from build123d import *

# Parameters (mm, degrees)
CHAMFER1_SIZE = 0.2


with BuildPart() as part:
    # Sketch1 → Revolve1 (revolve)
    with BuildSketch(Plane.XY, mode=Mode.PRIVATE) as revolve1_sk:
        Polygon((2.52, 0), (2.52, 4), (3.05, 4), (3.05, 6.4), (4.05, 6.4), (4.05, 4), (3.05, 0), align=None)
    revolve(revolve1_sk.sketch.rotate(Axis((0, 0, 0), (0, 1, 0)), 90), axis=Axis((0, 0, 0), (0, 1, 0)))

    # Chamfer1
    chamfer1_edges = [part.edges().sort_by_distance(p)[0] for p in [
        (0, 6.4, 3.05),
    ]]
    chamfer(chamfer1_edges, length=CHAMFER1_SIZE)


solid = part.part
Verification items for the finished model (mm, model axes). A direction names the side the tool comes from. Give positions to 0.01 mm unless a question says otherwise; leave off trailing zeros. Write each loop counter-clockwise with the first axis right and the second up, starting at its lowest first coordinate (ties: lowest second). Pieces come first, ordered by that corner, then holes. Notation, with made-up numbers: (59.5, 87) - (103.5, 87) arc R36 ccw to (103.5, 121) - close; hole circle Ø4 at (89.25, -13.75). An arc over 180 degrees is marked (long way). Answer as CSV lines item,"result". Start each with the question number.
1. Sectioned sample at D-D (y = 5). Record the boundary of the cut face in (x, z).
2. Depth check by flat-ended pin: pin 1 (1 mm diameter, centred on y = 1, z = -3, fed in from -X); pin 2 (2 mm diameter, centred on y = 5, z = 0.5, fed in from +X); pin 3 (1 mm diameter, centred on x = -1, y = 2, fed in from +Z); pin 4 (1.5 mm diameter, centred on x = -1.5, y = 2, fed in from -Z). Enter the tip coordinate at first touch or a pass-through.
3. Thickness scan on line 1 (X direction, y = 5.65, z = 0); line 2 (Z direction, x = 1, y = 2.75); line 3 (Y direction, x = 1.5, z = 2.5). Record the ranges inside material, lowest first.
4. Sectioned sample at A-A (x = 0). Record the boundary of the cut face in (y, z), then the cut area to 3 significant figures.
5. Draft check along Z on faces 1 (the face through (-2, 0, 2)), 2 (the face through (1.856, 5.115, 2.42)), 3 (the face through (3.24, 1.08, 0.72)), 4 (the face through (1.53, 2.03, 2)). Enter one of: pulls with the +Z half, pulls with the -Z half, needs draft (parallel to the pull), parting line crosses it, or undercut.
6. Set-up check for faces 5 (the face through (-2, 4, -2)), 6 (the face through (2, 6.4, -3)): record each of +Z, -Z, +X, -X, +Y, -Y from which the full face is reachable in a straight line by a thin tool's end or side.
7. Sectioned sample at C-C (y = 1). Record the boundary of the cut face in (x, z), then the cut area to 3 significant figures.
8. Sectioned sample at B-B (z = 0). Record the boundary of the cut face in (x, y), then the cut area to 3 significant figures.
Derived:
1,outline,"circle Ø8.1 at (0, 0); hole circle Ø6.1 at (0, 0)"
2,pin 1,"x = -2.18"
2,pin 2,"x = 4.05"
2,pin 3,"z = 3.58"
2,pin 4,"z = -3.55"
3,line 1,"-4.05 to -3.05, 3.05 to 4.05"
3,line 2,"-3.6 to -2.31, 2.31 to 3.6"
3,line 3,"0 to 4"
4,outline,"(0, -3.05) - (4, -4.05) - (6.4, -4.05) - (6.4, -3.25) - (6.2, -3.05) - (4, -3.05) - (4, -2.52) - (0, -2.52) - close; (0, 2.52) - (4, 2.52) - (4, 3.05) - (6.2, 3.05) - (6.4, 3.25) - (6.4, 4.05) - (4, 4.05) - (0, 3.05) - close"
4,area,"13.0 mm²"
5,face 1,"needs draft"
5,face 2,"undercut"
5,face 3,"parting line crosses it"
5,face 4,"undercut"
6,face 5,"+Y"
6,face 6,"+Z, -Z, +X, -X, +Y"
7,outline,"circle Ø6.6 at (0, 0); hole circle Ø5.04 at (0, 0)"
7,area,"14.3 mm²"
8,outline,"(-4.05, 4) - (-3.05, 0) - (-2.52, 0) - (-2.52, 4) - (-3.05, 4) - (-3.05, 6.2) - (-3.25, 6.4) - (-4.05, 6.4) - close; (2.52, 0) - (3.05, 0) - (4.05, 4) - (4.05, 6.4) - (3.25, 6.4) - (3.05, 6.2) - (3.05, 4) - (2.52, 4) - close"
8,area,"13.0 mm²"
